Design review of the part built by this model. Coordinates are the model's own, in mm. A direction names the side the tool comes from. Round coordinates to 2 decimals unless told otherwise and drop trailing zeros. Loops run counter-clockwise (first coordinate to the right, second up) from the corner with the lowest first, then second, coordinate; pieces in that order, holes last. Notation, with made-up numbers: M 3.25,-29 L 62.25,-29 A15 cw 62.25,-1 Z; hole C -1,87 d8. An arc over 180 degrees is marked long. One line per item, written item: value. Start each with the question number.
Item 1: We need section B-B (x = -9). Write out the cut boundary in (y, z).
Item 2: For line 1 along Z through (x, y) = (2, 2.6); line 2 along Z through (x, y) = (2.5, 0.3); line 3 along X through (y, z) = (0.6, -12), list the stretches that pass through material, from the lowest coordinate up.
Item 3: We need section A-A (z = -12). Write out the cut boundary in (x, y), then the cut area to 3 significant figures.
Item 4: We need section D-D (x = 6.5). Write out the cut boundary in (y, z), then the cut area to 3 significant figures.
Item 5: For faces 3 (the cylindrical face through (-12.926, 1.479, 5.826)), 4 (the flat face through (-15, 2, 13.722)), list the 3-axis set-ups (+Z, -Z, +X, -X, +Y, -Y) from which the entire face can be reached by the end or side of a thin tool; tool diameter is ignored.
Item 6: Mouldability with a two-part tool opening along Z and no side actions: class faces 1 (the flat face through (4, 2, -15.957)), 2 (the flat face through (22.6, 1.5, -13.3)) as released by +Z, released by -Z, zero draft, split by the parting line, or undercut.
Item 7: Clearance check with flat-ended pins moving along their axes: pin 1 (1.1 mm diameter, centred on y = 1.5, z = 0, fed in from -X); pin 2 (1.1 mm diameter, centred on y = 1.5, z = -16.5, fed in from -X); pin 3 (1 mm diameter, centred on y = 1, z = 1.5, fed in from +X). State where each tip first meets the part, or that it passes through.
Item 8: We need section C-C (y = 2.25). State how many separate pieces and enclosed holes the cut face has, then the cut area to 3 significant figures.
from build123d import *

# Parameters (mm, degrees)
BOSS_EXTRUDE1_DEPTH = 3
CUT_EXTRUDE1_DEPTH  = 4


with BuildPart() as part:
    # Sketch1 → Boss-Extrude1 (new body)
    with BuildSketch(Plane(origin=(0, 0, 0), x_dir=(1, 0, 0), z_dir=(0, 1, 0))):
        with BuildLine():
            Line((-6.037453791, -13.924683413), (-12.047861431, -7.914275773))
            ThreePointArc((-12.047861431, -7.914275773), (-12.926541087, -5.792955429), (-12.047861431, -3.671635086))
            Line((-12.047861431, -3.671635086), (8.458235223, 16.834461569))
            ThreePointArc((8.458235223, 16.834461569), (10.579555567, 17.713141225), (12.700875911, 16.834461569))
            Line((12.700875911, 16.834461569), (18.711283551, 10.824053929))
            ThreePointArc((18.711283551, 10.824053929), (19.418390332, 10.53116071), (20.125497113, 10.824053929))
            Line((20.125497113, 10.824053929), (25.075244581, 15.773801397))
            Line((25.075244581, 15.773801397), (17.606467502, 23.242578477))
            ThreePointArc((17.606467502, 23.242578477), (15.984350757, 24.326442233), (14.070933596, 24.707044571))
            Line((14.070933596, 24.707044571), (7.088177538, 24.707044571))
            ThreePointArc((7.088177538, 24.707044571), (5.174760376, 24.326442233), (3.552643632, 23.242578477))
            Line((3.552643632, 23.242578477), (-18.455978339, 1.233956505))
            ThreePointArc((-18.455978339, 1.233956505), (-19.539842096, -0.388160239), (-19.920444433, -2.301577401))
            Line((-19.920444433, -2.301577401), (-19.920444433, -9.284333458))
            ThreePointArc((-19.920444433, -9.284333458), (-19.539842096, -11.19775062), (-18.455978339, -12.819867364))
            Line((-18.455978339, -12.819867364), (-10.987201259, -20.288644444))
            Line((-10.987201259, -20.288644444), (-6.037453791, -15.338896975))
            ThreePointArc((-6.037453791, -15.338896975), (-5.744560572, -14.631790194), (-6.037453791, -13.924683413))
        make_face()
    extrude(amount=BOSS_EXTRUDE1_DEPTH)

    # Sketch2 → Cut-Extrude1 (cut, through all)
    with BuildSketch(Plane(origin=(0, 3, 0), x_dir=(1, 0, 0), z_dir=(0, 1, 0))):
        Polygon((-15.670444433, 2.136481822), (-15.670444433, 0.336481822), (-14.320444433, 0.336481822), (-14.320444433, -1.013518178), (-12.520444433, -1.013518178), (-12.520444433, 0.336481822), (-11.170444433, 0.336481822), (-11.170444433, 2.136481822), (-12.520444433, 2.136481822), (-12.520444433, 3.486481822), (-14.320444433, 3.486481822), (-14.320444433, 2.136481822), align=None)
        Polygon((-12.520444433, -10.572392681), (-14.320444433, -10.572392681), (-14.320444433, -11.922392681), (-15.670444433, -11.922392681), (-15.670444433, -13.722392681), (-14.320444433, -13.722392681), (-14.320444433, -15.072392681), (-12.520444433, -15.072392681), (-12.520444433, -13.722392681), (-11.170444433, -13.722392681), (-11.170444433, -11.922392681), (-12.520444433, -11.922392681), align=None)
        Polygon((18.508992818, 17.307044571), (19.858992818, 17.307044571), (19.858992818, 19.107044571), (18.508992818, 19.107044571), (18.508992818, 20.457044571), (16.708992818, 20.457044571), (16.708992818, 19.107044571), (15.358992818, 19.107044571), (15.358992818, 17.307044571), (16.708992818, 17.307044571), (16.708992818, 15.957044571), (18.508992818, 15.957044571), align=None)
        Polygon((36.829555567, -13.722392681), (36.829555567, -11.922392681), (35.479555567, -11.922392681), (35.479555567, -10.572392681), (33.679555567, -10.572392681), (33.679555567, -11.922392681), (32.329555567, -11.922392681), (32.329555567, -13.722392681), (33.679555567, -13.722392681), (33.679555567, -15.072392681), (35.479555567, -15.072392681), (35.479555567, -13.722392681), align=None)
        Polygon((5.800118315, 19.107044571), (4.450118315, 19.107044571), (4.450118315, 20.457044571), (2.650118315, 20.457044571), (2.650118315, 19.107044571), (1.300118315, 19.107044571), (1.300118315, 17.307044571), (2.650118315, 17.307044571), (2.650118315, 15.957044571), (4.450118315, 15.957044571), (4.450118315, 17.307044571), (5.800118315, 17.307044571), align=None)
        Polygon((36.829555567, 2.136481822), (35.479555567, 2.136481822), (35.479555567, 3.486481822), (33.679555567, 3.486481822), (33.679555567, 2.136481822), (32.329555567, 2.136481822), (32.329555567, 0.336481822), (33.679555567, 0.336481822), (33.679555567, -1.013518178), (35.479555567, -1.013518178), (35.479555567, 0.336481822), (36.829555567, 0.336481822), align=None)
        Polygon((4.450118315, -32.042955429), (4.450118315, -30.692955429), (5.800118315, -30.692955429), (5.800118315, -28.892955429), (4.450118315, -28.892955429), (4.450118315, -27.542955429), (2.650118315, -27.542955429), (2.650118315, -28.892955429), (1.300118315, -28.892955429), (1.300118315, -30.692955429), (2.650118315, -30.692955429), (2.650118315, -32.042955429), align=None)
        Polygon((18.508992818, -32.042955429), (18.508992818, -30.692955429), (19.858992818, -30.692955429), (19.858992818, -28.892955429), (18.508992818, -28.892955429), (18.508992818, -27.542955429), (16.708992818, -27.542955429), (16.708992818, -28.892955429), (15.358992818, -28.892955429), (15.358992818, -30.692955429), (16.708992818, -30.692955429), (16.708992818, -32.042955429), align=None)
    extrude(amount=-CUT_EXTRUDE1_DEPTH, mode=Mode.SUBTRACT)


solid = part.part
A:
1. outline: M 0,-10.69 L 3,-10.69 L 3,0.62 L 0,0.62 Z; M 0,10.96 L 3,10.96 L 3,18.3 L 0,18.3 Z
2. line 1: -21.69 to -19.11, -17.31 to -10.38
2. line 2: -22.19 to -19.11, -17.31 to -10.88
2. line 3: -7.69 to 3.62, 17.54 to 21.3
3. outline: M -7.69,0 L 3.62,0 L 3.62,3 L -7.69,3 Z; M 17.54,0 L 21.3,0 L 21.3,3 L 17.54,3 Z
3. area: 45.2 mm2
4. outline: M 0,-24.67 L 3,-24.67 L 3,-14.88 L 0,-14.88 Z
4. area: 29.4 mm2
5. face 3: +X, +Y, -Y
5. face 4: +Y, -Y
6. face 1: undercut
6. face 2: released by +Z
7. pin 1: x = -19.6
7. pin 2: x = -3.74
7. pin 3: x = -9.38
8. separate pieces: 1
8. enclosed holes: 4
8. area: 496 mm2
